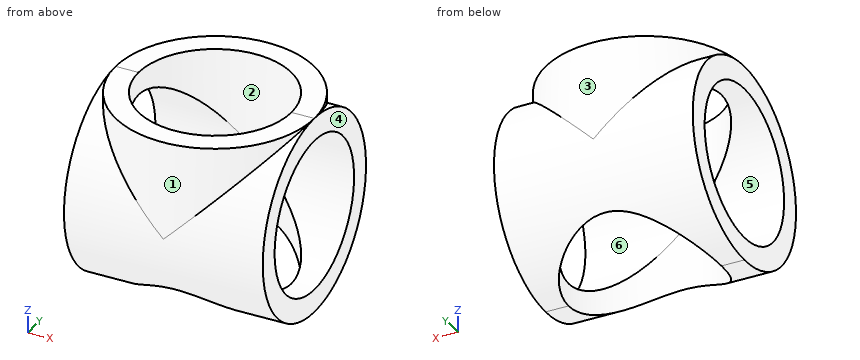
from build123d import *
from build123d.topology import SkipClean

# Parameters (mm, degrees)
BOSS_EXTRUDE4_DEPTH      = 13
BOSS_EXTRUDE4_DEPTH_BACK = 13
SKETCH46_R               = 13
SKETCH47_R               = 13
BOSS_EXTRUDE5_DEPTH      = 13
SKETCH48_R               = 10
CUT_EXTRUDE1_DEPTH       = 33
SKETCH49_R               = 10
CUT_EXTRUDE2_DEPTH       = 33


with BuildPart() as part:
    # Sketch46 → Boss-Extrude4 (new, two sides: drawn at the far end of the back side and taken through both)
    with BuildSketch(Plane(origin=(0, 0, 0), x_dir=(0, 0, -1), z_dir=(1, 0, 0)).offset(-BOSS_EXTRUDE4_DEPTH_BACK)):
        Circle(SKETCH46_R)
    extrude(amount=BOSS_EXTRUDE4_DEPTH + BOSS_EXTRUDE4_DEPTH_BACK)

    # Sketch47 → Boss-Extrude5 (add)
    with SkipClean():  # the faces are left unmerged after this step: merging them gives an invalid solid
        with BuildSketch(Plane.XY):
            Circle(SKETCH47_R)
        extrude(amount=BOSS_EXTRUDE5_DEPTH)

    # Sketch48 → Cut-Extrude1 (cut)
    with SkipClean():  # the faces are left unmerged after this step: merging them gives an invalid solid
        with BuildSketch(Plane.XY.offset(13)):
            Circle(SKETCH48_R)
        extrude(amount=-CUT_EXTRUDE1_DEPTH, mode=Mode.SUBTRACT)

    # Sketch49 → Cut-Extrude2 (cut)
    with SkipClean():  # the faces are left unmerged after this step: merging them gives an invalid solid
        with BuildSketch(Plane.ZY.offset(13)):
            Circle(SKETCH49_R)
        extrude(amount=-CUT_EXTRUDE2_DEPTH, mode=Mode.SUBTRACT)


solid = part.part
Read the model definition and answer for the solid it produces. Units are mm, in the model's axes. Face numbers are marked on the shaded views. A direction names the side the tool comes from. Coordinates: 2 decimals unless noted, no trailing zeros. Write each loop counter-clockwise with the first axis right and the second up, starting at its lowest first coordinate (ties: lowest second). Pieces come first, ordered by that corner, then holes. Notation, with made-up numbers: (44, -25.5) -> (70, -25.5) arc R23 ccw to (70, -9.5) -> close; hole circle Ø1 at (-13, 72.25). An arc over 180 degrees is marked (long way). Return JSON: item names as keys, results as strings.
(1) For a pull along Z with two mould halves and no side action, classify the marked faces 4, 5 and 6 as pulls with the +Z half, pulls with the -Z half, needs draft (parallel to the pull), parting line crosses it, or undercut.
Answers below:
{"face 4": "needs draft", "face 5": "undercut", "face 6": "undercut"}
(2) The part is cut by section B-B on z = 3. Give the vertices of the cut face in (x, y).
Answers below:
{"outline": "(-13, -12.65) -> (-3, -12.65) arc R13 ccw to (3, -12.65) -> (13, -12.65) -> (13, -9.54) -> (3, -9.54) arc R10 cw to (-3, -9.54) -> (-13, -9.54) -> close; (-13, 9.54) -> (-3, 9.54) arc R10 cw to (3, 9.54) -> (13, 9.54) -> (13, 12.65) -> (3, 12.65) arc R13 ccw to (-3, 12.65) -> (-13, 12.65) -> close"}
(3) The part is cut by section D-D on z = -8.5. Give the vertices of the cut face in (x, y), then the cut area to 3 significant figures.
Answers below:
{"outline": "(-13, -9.84) -> (-1.8, -9.84) arc R10 cw to (-8.5, -5.27) -> (-13, -5.27) -> close; (-13, 5.27) -> (-8.5, 5.27) arc R10 cw to (-1.8, 9.84) -> (-13, 9.84) -> close; (1.8, -9.84) -> (13, -9.84) -> (13, -5.27) -> (8.5, -5.27) arc R10 cw to start; (1.8, 9.84) arc R10 cw to (8.5, 5.27) -> (13, 5.27) -> (13, 9.84) -> close", "area": "125 mm^2"}
(4) Consider line 1 along Y through (x, z) = (-3.5, 0); line 2 along X through (y, z) = (7, 8.5); line 3 along Z through (x, y) = (10.5, 8.5). Determine where each line is inside the solid, lowest interval first. Write a range as from..to.
Answers below:
{"line 1": "-13..-10, 10..13", "line 2": "-13..-7.14, 7.14..13", "line 3": "-9.84..-5.27, 5.27..9.84"}
(5) The part is cut by section A-A on y = 2. Give the vertices of the cut face in (x, z), then the cut area to 3 significant figures.
Answers below:
{"outline": "(-13, -12.85) -> (-9.8, -12.85) -> (-9.8, -9.8) -> (-13, -9.8) -> close; (-13, 9.8) -> (-9.8, 9.8) -> (-9.8, 13) -> (-12.85, 13) -> (-12.85, 12.85) -> (-13, 12.85) -> close; (9.8, -12.85) -> (13, -12.85) -> (13, -9.8) -> (9.8, -9.8) -> close; (9.8, 9.8) -> (13, 9.8) -> (13, 12.85) -> (12.85, 12.85) -> (12.85, 13) -> (9.8, 13) -> close", "area": "40.0 mm^2"}
(6) The part is cut by section C-C on x = 2. Give the vertices of the cut face in (y, z).
Answers below:
{"outline": "(-12.85, 2) arc R13 ccw to (-9.8, -8.54) -> (-9.8, -2) arc R10 cw to (-9.8, 2) -> (-9.8, 13) -> (-12.85, 13) -> close; (9.8, -8.54) arc R13 ccw to (12.85, 2) -> (12.85, 13) -> (9.8, 13) -> (9.8, 2) arc R10 cw to (9.8, -2) -> close"}
(7) Which of the six approach directions +Z, -Z, +X, -X, +Y, -Y give full straight-line access (tool end or side, diameter ignored) to the marked faces 1, 2 and 3?
Answers below:
{"face 1": "+Z, -Y", "face 2": "+Z, -Z", "face 3": "+Z, +Y"}
